Autodesk Inventor part; units mm, degrees
ref_plane "Work Plane1" through (0, 0, 5) normal (0, 0, 1) x (1, 0, 0)
ref_plane "Work Plane3" through (5, 0, 0) normal (1, 0, 0) x (0, 1, 0)
ref_plane "XZ Plane" through (0, 0, 0) normal (0, 1, 0) x (-1, 0, 0)
sketch "Sketch1" plane through (0, 0, 0) normal (0, 1, 0) x (-1, 0, 0)
  circle A0 centre (0, 0) radius 5
  dimension "d0" = 10
extrude "Extrusion1" add sketch "Sketch1" along normal blind 45
ref_plane "Work Plane1" through (0, 0, 5) normal (0, 0, 1) x (1, 0, 0)
sketch "Sketch2" plane through (0, 0, 5) normal (0, 0, 1) x (1, 0, 0)
  point P0 (0, 0)
  point P1 (0, 7)
  dimension "d3" = 7
hole "Hole1" at (0, 7, 5) direction (0, 0, -1) diameter 3.302 end through all countersink diameter 8 countersink angle 90
sketch "Sketch5" plane through (0, 45, 0) normal (0, 1, 0) x (1, 0, 0)
  line L0 (-5, 5) -> (-1.5, 5)
  line L1 (-1.5, 5) -> (-1.5, -5)
  line L2 (-1.5, -5) -> (-5, -5)
  line L3 (-5, -5) -> (-5, 5)
  line L4 (1.5, 5) -> (5, 5)
  line L5 (5, 5) -> (5, -5)
  line L6 (5, -5) -> (1.5, -5)
  line L7 (1.5, -5) -> (1.5, 5)
  point P0 (0, 0)
  point P1 (-5, 0)
  point P2 (1.5, 0)
  point P3 (5, 0)
  point P4 (-1.5, 0)
  dimension "d16" = 3
  dimension "d17" = 10
  dimension "d18" = 10
  dimension "d27" = 5
extrude "Extrusion2" cut sketch "Sketch5" against normal blind 17
sketch "Sketch6" plane through (1.5, 45, 4.7697) normal (1, 0, 0) x (0, 0, -1)
  circle A0 centre (4.7697, -4) radius 1
  line L0 (0, 0) -> (9.5394, 0)
  line L1 (0, -17) -> (0, 0)
  line L2 (0, -17) -> (9.5394, -17)
  line L3 (9.5394, 0) -> (0, 0)
  line L4 (9.5394, 0) -> (9.5394, -17)
  line L5 (4.7697, 0) -> (4.7697, -17)
  point P0 (4.7697, -45)
  dimension "d32" = 2
  dimension "d33" = 4
hole "Hole2" at (1.5, 41, 0) direction (-1, 0, 0) diameter 2 end through all
ref_plane "Work Plane3" through (5, 0, 0) normal (1, 0, 0) x (0, 1, 0)
sketch "Sketch10" plane through (5, 0, 0) normal (1, 0, 0) x (0, 1, 0)
  arc A0 (39.5485, -3.7274) -> (45, 0) centre (41, 0) ccw
  circle A1 centre (41, 0) radius 1
  line L0 (28, 0.7697) -> (39.5485, -3.7274)
  line L1 (28, 4.7697) -> (28, -4.7697)
  line L2 (28, 4.7697) -> (45, 4.7697)
  line L3 (45, -5) -> (45, -4.7697)
  line L4 (34, -5) -> (45, -5)
  line L5 (45, 4.7697) -> (45, 5)
  line L6 (45, -5) -> (45, 5)
  line L7 (45, 5) -> (39.1833, 5)
  line L8 (39.1833, 5) -> (42.4515, 3.7274)
  line L9 (45, 4.7697) -> (28, 4.7697)
  line L10 (0, 5) -> (45, 5)
  line L11 (34, -5) -> (35.1609, -2.0188)
  arc A2 (45, 0) -> (42.4515, 3.7274) centre (41, 0) ccw
  point P0 (0, 0)
  point P1 (45, -4.7697)
  dimension "d54" = 8
  dimension "d55" = 6
  dimension "d56" = 4
extrude "Extrusion3" cut sketch "Sketch10" against normal through all contours A0 L6 L3 L4 L11 L0 | A2 L8 L2 L6 | L2 L8 L7 L5
chamfer "Chamfer1" distance 2 angle 45 1 edges at (-0.2563, 8.631, -4.9934)
properties part number "barrel_hinge-male" material "Stainless Steel"
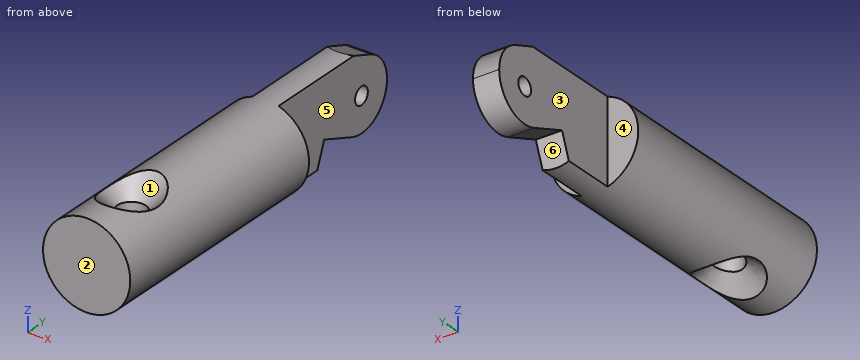
Geometry check sheet. Reference: the model listing, model coordinates, mm. Face numbers are marked on the shaded views. A direction names the side the tool comes from. Round coordinates to 2 decimals unless told otherwise and drop trailing zeros. Loops run counter-clockwise (first coordinate to the right, second up) from the corner with the lowest first, then second, coordinate; pieces in that order, holes last. Notation, with made-up numbers: (43, 24.25) - (65, 24.25) arc R30 cw to (65, 51.25) - close; hole circle Ø2 at (89.25, 88). An arc over 180 degrees is marked (long way). Use a Markdown table: item, result.
Q1. Draft check along X on the marked faces 1, 2 and 3. Enter one of: released by +X, released by -X, zero draft, split by the parting line, or undercut.
Solutions:
| item | result |
|---|---|
| face 1 | undercut |
| face 2 | zero draft |
| face 3 | released by -X |
Q2. Material ranges on line 1 (Y direction, x = 0, z = 0); line 2 (Z direction, x = 0.3, y = 41); line 3 (Y direction, x = 0.25, z = 1.75), recorded low to high.
Solutions:
| item | result |
|---|---|
| line 1 | y = 0 to 5.35, 8.65 to 40, 42 to 45 |
| line 2 | z = -4 to -1, 1 to 4.29 |
| line 3 | y = 0 to 5.37, 8.63 to 44.6 |
Q3. Cross-section at B-B on x = 0. State how many separate pieces and enclosed holes the cut face has, plus the area to 3 significant figures.
Solutions:
| item | result |
|---|---|
| separate pieces | 2 |
| enclosed holes | 1 |
| area | 376 mm2 |
Q4. Access from +Z, -Z, +X, -X, +Y, -Y to the whole of each face (thin tool, end or side, straight path). Record for the marked faces 4, 5 and 6.
Solutions:
| item | result |
|---|---|
| face 4 | +Z, -Z, -X, +Y |
| face 5 | +Z, -Z, +X, +Y |
| face 6 | -Z, +X, -X |
Q5. Cross-section at C-C on y = 12. Record the cut outline in (x, z).
Solutions:
| item | result |
|---|---|
| outline | circle Ø10 at (0, 0) |
Q6. Go/stop test with flat-tipped pins: P1, Ø3, axis at x = -3.5, y = 9, coming from the -Z side; P2, Ø3, axis at x = 2.5, z = -2, coming from the +Y side; P3, Ø2, axis at y = 36.5, z = 2.5, coming from the +X side. Record where each tip stops, or that it passes through.
Solutions:
| item | result |
|---|---|
| P1 | stops at z = -4.47 |
| P2 | stops at y = 44.9 |
| P3 | stops at x = 1.5 |
Q7. Cross-section at D-D on y = 31. Record the cut outline in (x, z).
Solutions:
| item | result |
|---|---|
| outline | (-1.5, -4.77) arc R5 ccw to (1.5, -4.77) - (1.5, 4.77) arc R5 ccw to (-1.5, 4.77) - close |
Q8. Cross-section at A-A on y = 41. Record the cut outline in (x, z).
Solutions:
| item | result |
|---|---|
| outline | (-1.5, -4) - (1.5, -4) - (1.5, -1) - (-1.5, -1) - close; (-1.5, 1) - (1.5, 1) - (1.5, 4.29) - (-1.5, 4.29) - close |
